from build123d import *

# Parameters (mm, degrees)
F1_DEPTH = 10
F2_R     = 1.5
F3_DEPTH = 10.001
F4_R     = 0.5


with BuildPart() as f1:
    # F0 (on Top) → F1 (new body)
    with BuildSketch(Plane.XY):
        Polygon((41.192254, 61.494219), (-28.807746, 61.494219), (-28.807746, -8.505781), (21.192254, -8.505781), (21.192254, 11.494219), (41.192254, 11.494219), align=None)
    extrude(amount=F1_DEPTH)

    # F2 (on Top) → F3 (cut, through all)
    with BuildSketch(Plane.XY):
        with Locations((-23.807746, 56.494219)):
            Circle(F2_R)
        with Locations((11.277618, 56.494219)):
            Circle(F2_R)
        with Locations((11.277618, 16.494219)):
            Circle(F2_R)
        with Locations((-23.807746, 16.494219)):
            Circle(F2_R)
    extrude(amount=F3_DEPTH, mode=Mode.SUBTRACT)

    # F4
    f4_edges = [f1.edges().sort_by_distance(p)[0] for p in [
        (-25.307746, 16.494219, 10),
        (-25.307746, 56.494219, 10),
        (9.777618, 56.494219, 10),
        (9.777618, 16.494219, 10),
    ]]
    fillet(f4_edges, radius=F4_R)


solid = f1.part
Build history of the part. All positions in model axes, mm. A direction names the side the tool comes from. Round coordinates to 2 decimals unless told otherwise and drop trailing zeros. Write each loop counter-clockwise with the first axis right and the second up, starting at its lowest first coordinate (ties: lowest second). Pieces come first, ordered by that corner, then holes. Notation, with made-up numbers: M -39,62 L -29,62 A31 ccw -29,97 Z; hole C 67,27.5 d11. An arc over 180 degrees is marked long. Use CSV: the item, a comma, the result in double quotes.
1. Saw through at A-A (z = 3.75). Give the cut face in (x, y).
Reply:
outline,"M -28.81,-8.51 L 21.19,-8.51 L 21.19,11.49 L 41.19,11.49 L 41.19,61.49 L -28.81,61.49 Z; hole C -23.81,16.49 d3; hole C -23.81,56.49 d3; hole C 11.28,16.49 d3; hole C 11.28,56.49 d3"
2. Two-plate mould, pull along X, no slides. Class faces 3 (the face through (31, 11.494, 5)), 4 (the face through (-28.808, 27, 5)), 5 (the face through (-24.13, 55.03, 4.68)): +X half, -X half, draft (parallel to the pull), parting line (faces both ways), or undercut.
Reply:
face 3,"draft"
face 4,"-X half"
face 5,"undercut"
3. Tool access for faces 1 (the face through (11.08, 17.98, 4.68)), 2 (the face through (21.192, 1, 5)): list every direction of +Z, -Z, +X, -X, +Y, -Y with a clear straight run to the whole face (end or side of a thin tool).
Reply:
face 1,"+Z, -Z"
face 2,"+Z, -Z, +X, -Y"
4. Saw through at B-B (y = 5.5). Give the cut face in (x, z), plus the area to 3 significant figures.
Reply:
outline,"M -28.81,0 L 21.19,0 L 21.19,10 L -28.81,10 Z"
area,"500 mm²"
5. Wall check: probe 1 along X at (y, z) = (15.5, 8.75); probe 2 along X at (y, z) = (56, 1.5); probe 3 along Y at (x, z) = (11, 5.75). Give the ranges that are in metal, low to high. Write a range as from..to.
Reply:
probe 1,"x = -28.81..-24.93, -22.68..10.15, 12.4..41.19"
probe 2,"x = -28.81..-25.22, -22.39..9.86, 12.69..41.19"
probe 3,"y = -8.51..15.02, 17.97..55.02, 57.97..61.49"
6. Saw through at C-C (x = 26.5). Give the cut face in (y, z), plus the area to 3 significant figures.
Reply:
outline,"M 11.49,0 L 61.49,0 L 61.49,10 L 11.49,10 Z"
area,"500 mm²"
7. Flat gauge pins, fed straight in: pin 1 (2 mm diameter, centred on x = 24.5, z = 9, fed in from -Y); pin 2 (2.5 mm diameter, centred on x = -23.81, y = 16.49, fed in from -Z). Where does each tip first touch, or does it go through?
Reply:
pin 1,"stops at y = 11.49"
pin 2,"passes through"
